Autodesk Inventor part; units mm, degrees
ref_plane "YZ Plane" through (0, 0, 0) normal (1, 0, 0) x (0, 1, 0)
ref_plane "XZ Plane" through (0, 0, 0) normal (0, 1, 0) x (-1, 0, 0)
ref_plane "XY Plane" through (0, 0, 0) normal (0, 0, 1) x (1, 0, 0)
sketch "Sketch1" plane through (0, 0, 0) normal (0, 1, 0) x (-1, 0, 0)
  line L0 (0, 0) -> (10, 0) construction
  circle A0 centre (10, 0) radius 3.75
  circle A1 centre (10, 0) radius 1.75
  line L1 (0, 0) -> (-10, 0) construction
  circle A2 centre (-10, 0) radius 4.25
  line L2 (10.0938, 3.7488) -> (-9.8938, 4.2487)
  line L3 (10.0938, -3.7488) -> (-9.8938, -4.2487)
  dimension "d1" = 7.5
  dimension "d0" = 10
  dimension "d2" = 3.5
  dimension "d3" = 10
extrude "Extrusion1" add sketch "Sketch1" along normal mid plane 3
sketch "Sketch2" plane through (0, 1.5, 0) normal (0, 1, 0) x (1, 0, 0)
  arc A0 (9.8938, -4.2487) -> (9.8938, 4.2487) centre (10, 0) ccw
  circle A1 centre (10, 0) radius 2.5
  circle A2 centre (10, 0) radius 4.25
  point P0 (0, 0)
  point P1 (9.8937, 4.2487)
  point P2 (9.8938, -4.2487)
  dimension "d9" = 5
extrude "Extrusion2" add sketch "Sketch2" along normal blind 1.5
sketch "Sketch4" plane through (10, 1.5, 0) normal (0, 1, 0) x (1, 0, 0)
  circle A0 centre (0, 0) radius 2.5
  circle A1 centre (0, 0) radius 2.5
  point P0 (-10, 0)
  dimension "d13" = 5
extrude "Extrusion3" cut sketch "Sketch4" against normal blind 1
sketch "Sketch5" plane through (10, 0.5, 0) normal (0, 1, 0) x (1, 0, 0)
  circle A0 centre (0, 0) radius 2.5
  circle A1 centre (0, 0) radius 1.25
  point P0 (-10, 0)
  dimension "d16" = 2.5
extrude "Extrusion4" cut sketch "Sketch5" against normal blind 0.8 contours A1
sketch "Sketch6" plane through (0, -1.5, 0) normal (0, -1, 0) x (1, 0, 0)
  arc A0 (9.8938, -4.2487) -> (9.8938, 4.2487) centre (10, 0) ccw
  circle A1 centre (10, 0) radius 2.5
  point P0 (0, 0)
  dimension "d19" = 5
extrude "Extrusion5" cut sketch "Sketch6" against normal blind 1.2
properties part number "eje de servo 1"
The model under review builds one solid part; all positions refer to its coordinate system, in mm. A direction names the side the tool comes from. Coordinates: 2 decimals unless noted, no trailing zeros. Loops run counter-clockwise (first coordinate to the right, second up) from the corner with the lowest first, then second, coordinate; pieces in that order, holes last. Notation, with made-up numbers: (57, 74.25) -> (104, 74.25) arc R26 ccw to (104, 102.25) -> close; hole circle Ø4 at (87.5, -25). An arc over 180 degrees is marked (long way). Use a Markdown table: item, result. Add a question column.
1. Machinability: for faces 1 (the face through (8.75, 0.11, -0.05)), 2 (the face through (9, -0.3, -1)), 3 (the face through (12, 3, 2)), 4 (the face through (5.75, 2.24, 0.09)), 5 (the face through (7.5, 1.7, 0.1)), which of the approach directions +Z, -Z, +X, -X, +Y, -Y give a long, thin tool a straight path to every point of the face, cutting with its end or side? Answer none if there is none.
2. Clearance check with flat-ended pins moving along their axes: pin 1 Ø3 at (x, z) = (10, 0) entering from +Y; pin 2 Ø2.5 at (x, z) = (-4, -1.5) entering from +Y; pin 3 Ø2 at (x, y) = (-8, 0.5) entering from -Z. State where each tip first meets the part, or that it passes through.
3. Draft analysis for pull direction Z (two halves, no side actions). For faces 6 (the face through (14.25, -0.02, -0.09)), 7 (the face through (0, -1.5, 0)), 8 (the face through (9, 0.5, 1)), state which applies: pulls with the +Z half, pulls with the -Z half, needs draft (parallel to the pull), parting line crosses it, or undercut.
4. Add section B-B on z = 3.5. Write out the cut boundary in (x, y), plus the area to 3 significant figures.
5. Add section A-A on z = 0. Write out the cut boundary in (x, y), plus the area to 4 significant figures.
6. To check wall thickness, follow line 1 (Z direction, x = -10, y = -0.45); line 2 (Z direction, x = 10, y = -0.1); line 3 (X direction, y = -0.9, z = -1.5). State the ranges of each line that lie inside material, in increasing order.
7. Add section C-C on x = 8.25. Write out the cut boundary in (y, z).
8. Add section D-D on z = -2. Write out the cut boundary in (x, y), plus the area to 3 significant figures.
Returned:
| question | item | result |
|---|---|---|
| 1 | face 1 | +Y, -Y |
| 1 | face 2 | -Y |
| 1 | face 3 | +Z, -Z, +X, -X, +Y |
| 1 | face 4 | -X, +Y |
| 1 | face 5 | +Y |
| 2 | pin 1 | stops at y = 0.5 |
| 2 | pin 2 | stops at y = 1.5 |
| 2 | pin 3 | stops at z = -3.83 |
| 3 | face 6 | parting line crosses it |
| 3 | face 7 | needs draft |
| 3 | face 8 | undercut |
| 4 | outline | (-11.35, -1.5) -> (12.41, -1.5) -> (12.41, 3) -> (7.59, 3) -> (7.59, 1.5) -> (-11.35, 1.5) -> close |
| 4 | area | 78.5 mm² |
| 5 | outline | (-13.75, -1.5) -> (-11.75, -1.5) -> (-11.75, 1.5) -> (-13.75, 1.5) -> close; (-8.25, -1.5) -> (7.5, -1.5) -> (7.5, -0.3) -> (8.75, -0.3) -> (8.75, 0.5) -> (7.5, 0.5) -> (7.5, 3) -> (5.75, 3) -> (5.75, 1.5) -> (-8.25, 1.5) -> close; (11.25, -0.3) -> (12.5, -0.3) -> (12.5, -1.5) -> (14.25, -1.5) -> (14.25, 3) -> (12.5, 3) -> (12.5, 0.5) -> (11.25, 0.5) -> close |
| 5 | area | 65.75 mm² |
| 6 | line 1 | z = -3.75 to -1.75, 1.75 to 3.75 |
| 6 | line 2 | z = -4.25 to -1.25, 1.25 to 4.25 |
| 6 | line 3 | x = -13.44 to -10.9, -9.1 to 8, 12 to 13.98 |
| 7 | outline | (-1.5, -4.21) -> (1.5, -4.21) -> (1.5, -3.87) -> (3, -3.87) -> (3, -1.79) -> (0.5, -1.79) -> (0.5, 1.79) -> (3, 1.79) -> (3, 3.87) -> (1.5, 3.87) -> (1.5, 4.21) -> (-1.5, 4.21) -> (-1.5, 1.79) -> (-0.3, 1.79) -> (-0.3, -1.79) -> (-1.5, -1.79) -> close |
| 8 | outline | (-13.17, -1.5) -> (8.5, -1.5) -> (8.5, -0.3) -> (11.5, -0.3) -> (11.5, -1.5) -> (13.75, -1.5) -> (13.75, 3) -> (11.5, 3) -> (11.5, 0.5) -> (8.5, 0.5) -> (8.5, 3) -> (6.25, 3) -> (6.25, 1.5) -> (-13.17, 1.5) -> close |
| 8 | area | 80.9 mm² |
